```python
from build123d import *

# Parameters (mm, degrees)
BOSS_EXTRUDE1_DEPTH = 20.0000108


with BuildPart() as part:
    # Sketch1 → Boss-Extrude1 (new body)
    with BuildSketch(Plane(origin=(0, 0, 0), x_dir=(1, 0, 0), z_dir=(0, 1, 0))):
        with BuildLine():
            Line((-1.159549536, 2.070936998), (-3.090908521, 3.791368499))
            ThreePointArc((-3.090908521, 3.791368499), (-3.125119474, 3.931396235), (-3.006433754, 4.0132))
            Line((-3.006433754, 4.0132), (-1.7526, 4.0132))
            ThreePointArc((-1.7526, 4.0132), (-1.572994878, 4.087594878), (-1.4986, 4.2672))
            Line((-1.4986, 4.2672), (-1.4986, 4.7498))
            ThreePointArc((-1.4986, 4.7498), (-1.572994878, 4.929405122), (-1.7526, 5.0038))
            Line((-1.7526, 5.0038), (-4.7498, 5.0038))
            ThreePointArc((-4.7498, 5.0038), (-4.929405122, 4.929405122), (-5.0038, 4.7498))
            Line((-5.0038, 4.7498), (-5.0038, 1.7526))
            ThreePointArc((-5.0038, 1.7526), (-4.929405122, 1.572994878), (-4.7498, 1.4986))
            Line((-4.7498, 1.4986), (-4.2672, 1.4986))
            ThreePointArc((-4.2672, 1.4986), (-4.087594878, 1.572994878), (-4.0132, 1.7526))
            Line((-4.0132, 1.7526), (-4.0132, 3.006433754))
            ThreePointArc((-4.0132, 3.006433754), (-3.931396235, 3.125119474), (-3.791368499, 3.090908521))
            Line((-3.791368499, 3.090908521), (-2.070936998, 1.159549536))
            ThreePointArc((-2.070936998, 1.159549536), (-2.023228558, 1.08099247), (-2.0066, 0.9906))
            Line((-2.0066, 0.9906), (-2.0066, 0.7493))
            ThreePointArc((-2.0066, 0.7493), (-1.932205122, 0.569694878), (-1.7526, 0.4953))
            ThreePointArc((-1.7526, 0.4953), (-1.572994878, 0.420905122), (-1.4986, 0.2413))
            Line((-1.4986, 0.2413), (-1.4986, -0.2413))
            ThreePointArc((-1.4986, -0.2413), (-1.572994878, -0.420905122), (-1.7526, -0.4953))
            ThreePointArc((-1.7526, -0.4953), (-1.932205122, -0.569694878), (-2.0066, -0.7493))
            Line((-2.0066, -0.7493), (-2.0066, -0.9906))
            ThreePointArc((-2.0066, -0.9906), (-2.023228558, -1.08099247), (-2.070936998, -1.159549536))
            Line((-2.070936998, -1.159549536), (-3.791368499, -3.090908521))
            ThreePointArc((-3.791368499, -3.090908521), (-3.931396235, -3.125119474), (-4.0132, -3.006433754))
            Line((-4.0132, -3.006433754), (-4.0132, -1.7526))
            ThreePointArc((-4.0132, -1.7526), (-4.087594878, -1.572994878), (-4.2672, -1.4986))
            Line((-4.2672, -1.4986), (-4.7498, -1.4986))
            ThreePointArc((-4.7498, -1.4986), (-4.929405122, -1.572994878), (-5.0038, -1.7526))
            Line((-5.0038, -1.7526), (-5.0038, -4.7498))
            ThreePointArc((-5.0038, -4.7498), (-4.929405122, -4.929405122), (-4.7498, -5.0038))
            Line((-4.7498, -5.0038), (-1.7526, -5.0038))
            ThreePointArc((-1.7526, -5.0038), (-1.572994878, -4.929405122), (-1.4986, -4.7498))
            Line((-1.4986, -4.7498), (-1.4986, -4.2672))
            ThreePointArc((-1.4986, -4.2672), (-1.572994878, -4.087594878), (-1.7526, -4.0132))
            Line((-1.7526, -4.0132), (-3.006433754, -4.0132))
            ThreePointArc((-3.006433754, -4.0132), (-3.125119474, -3.931396235), (-3.090908521, -3.791368499))
            Line((-3.090908521, -3.791368499), (-1.159549536, -2.070936998))
            ThreePointArc((-1.159549536, -2.070936998), (-1.08099247, -2.023228558), (-0.9906, -2.0066))
            Line((-0.9906, -2.0066), (-0.7493, -2.0066))
            ThreePointArc((-0.7493, -2.0066), (-0.569694878, -1.932205122), (-0.4953, -1.7526))
            ThreePointArc((-0.4953, -1.7526), (-0.420905122, -1.572994878), (-0.2413, -1.4986))
            Line((-0.2413, -1.4986), (0.2413, -1.4986))
            ThreePointArc((0.2413, -1.4986), (0.420905122, -1.572994878), (0.4953, -1.7526))
            ThreePointArc((0.4953, -1.7526), (0.569694878, -1.932205122), (0.7493, -2.0066))
            Line((0.7493, -2.0066), (0.9906, -2.0066))
            ThreePointArc((0.9906, -2.0066), (1.08099247, -2.023228558), (1.159549536, -2.070936998))
            Line((1.159549536, -2.070936998), (3.090908521, -3.791368499))
            ThreePointArc((3.090908521, -3.791368499), (3.125119474, -3.931396235), (3.006433754, -4.0132))
            Line((3.006433754, -4.0132), (1.7526, -4.0132))
            ThreePointArc((1.7526, -4.0132), (1.572994878, -4.087594878), (1.4986, -4.2672))
            Line((1.4986, -4.2672), (1.4986, -4.7498))
            ThreePointArc((1.4986, -4.7498), (1.572994878, -4.929405122), (1.7526, -5.0038))
            Line((1.7526, -5.0038), (4.7498, -5.0038))
            ThreePointArc((4.7498, -5.0038), (4.929405122, -4.929405122), (5.0038, -4.7498))
            Line((5.0038, -4.7498), (5.0038, -1.7526))
            ThreePointArc((5.0038, -1.7526), (4.929405122, -1.572994878), (4.7498, -1.4986))
            Line((4.7498, -1.4986), (4.2672, -1.4986))
            ThreePointArc((4.2672, -1.4986), (4.087594878, -1.572994878), (4.0132, -1.7526))
            Line((4.0132, -1.7526), (4.0132, -3.006433754))
            ThreePointArc((4.0132, -3.006433754), (3.931396235, -3.125119474), (3.791368499, -3.090908521))
            Line((3.791368499, -3.090908521), (2.070936998, -1.159549536))
            ThreePointArc((2.070936998, -1.159549536), (2.023228558, -1.08099247), (2.0066, -0.9906))
            Line((2.0066, -0.9906), (2.0066, -0.7493))
            ThreePointArc((2.0066, -0.7493), (1.932205122, -0.569694878), (1.7526, -0.4953))
            ThreePointArc((1.7526, -0.4953), (1.572994878, -0.420905122), (1.4986, -0.2413))
            Line((1.4986, -0.2413), (1.4986, 0.2413))
            ThreePointArc((1.4986, 0.2413), (1.572994878, 0.420905122), (1.7526, 0.4953))
            ThreePointArc((1.7526, 0.4953), (1.932205122, 0.569694878), (2.0066, 0.7493))
            Line((2.0066, 0.7493), (2.0066, 0.9906))
            ThreePointArc((2.0066, 0.9906), (2.023228558, 1.08099247), (2.070936998, 1.159549536))
            Line((2.070936998, 1.159549536), (3.791368499, 3.090908521))
            ThreePointArc((3.791368499, 3.090908521), (3.931396235, 3.125119474), (4.0132, 3.006433754))
            Line((4.0132, 3.006433754), (4.0132, 1.7526))
            ThreePointArc((4.0132, 1.7526), (4.087594878, 1.572994878), (4.2672, 1.4986))
            Line((4.2672, 1.4986), (4.7498, 1.4986))
            ThreePointArc((4.7498, 1.4986), (4.929405122, 1.572994878), (5.0038, 1.7526))
            Line((5.0038, 1.7526), (5.0038, 4.7498))
            ThreePointArc((5.0038, 4.7498), (4.929405122, 4.929405122), (4.7498, 5.0038))
            Line((4.7498, 5.0038), (1.7526, 5.0038))
            ThreePointArc((1.7526, 5.0038), (1.572994878, 4.929405122), (1.4986, 4.7498))
            Line((1.4986, 4.7498), (1.4986, 4.2672))
            ThreePointArc((1.4986, 4.2672), (1.572994878, 4.087594878), (1.7526, 4.0132))
            Line((1.7526, 4.0132), (3.006433754, 4.0132))
            ThreePointArc((3.006433754, 4.0132), (3.125119474, 3.931396235), (3.090908521, 3.791368499))
            Line((3.090908521, 3.791368499), (1.159549536, 2.070936998))
            ThreePointArc((1.159549536, 2.070936998), (1.08099247, 2.023228558), (0.9906, 2.0066))
            Line((0.9906, 2.0066), (0.7493, 2.0066))
            ThreePointArc((0.7493, 2.0066), (0.569694878, 1.932205122), (0.4953, 1.7526))
            ThreePointArc((0.4953, 1.7526), (0.420905122, 1.572994878), (0.2413, 1.4986))
            Line((0.2413, 1.4986), (-0.2413, 1.4986))
            ThreePointArc((-0.2413, 1.4986), (-0.420905122, 1.572994878), (-0.4953, 1.7526))
            ThreePointArc((-0.4953, 1.7526), (-0.569694878, 1.932205122), (-0.7493, 2.0066))
            Line((-0.7493, 2.0066), (-0.9906, 2.0066))
            ThreePointArc((-0.9906, 2.0066), (-1.08099247, 2.023228558), (-1.159549536, 2.070936998))
        make_face()
    extrude(amount=BOSS_EXTRUDE1_DEPTH)


solid = part.part
```
The model under review builds one solid part; all positions refer to its coordinate system, in mm. A direction names the side the tool comes from. Give positions to 0.01 mm unless a question says otherwise; leave off trailing zeros. Loops run counter-clockwise (first coordinate to the right, second up) from the corner with the lowest first, then second, coordinate; pieces in that order, holes last. Notation, with made-up numbers: (22, -28) -> (58, -28) arc R11 ccw to (58, -21) -> close; hole circle Ø5 at (-38, 77.5). An arc over 180 degrees is marked (long way). Use CSV: the item, a comma, the result in double quotes.
1. To check wall thickness, follow probe 1 along Z at (x, y) = (2.25, 8.25); probe 2 along X at (y, z) = (15, -1); probe 3 along X at (y, z) = (3.75, -0.25). State the ranges of each line that lie inside material, in increasing order. Write a range as from..to.
Result:
probe 1,"z = -5..-4.01, -3.04..-1.36, 1.36..3.04, 4.01..5"
probe 2,"x = -2.01..2.01"
probe 3,"x = -1.5..1.5"
2. Consider section A-A, the plane x = -2.75. Write out the cut boundary in (y, z), then the cut area to 3 significant figures.
Result:
outline,"(0, -5) -> (20, -5) -> (20, -4.01) -> (0, -4.01) -> close; (0, -3.49) -> (20, -3.49) -> (20, -1.92) -> (0, -1.92) -> close; (0, 1.92) -> (20, 1.92) -> (20, 3.49) -> (0, 3.49) -> close; (0, 4.01) -> (20, 4.01) -> (20, 5) -> (0, 5) -> close"
area,"102 mm²"
3. Consider section C-C, the plane z = 2.5. Write out the cut boundary in (x, y) (3 decimals).
Result:
outline,"(-5.004, 0) -> (-4.013, 0) -> (-4.013, 20) -> (-5.004, 20) -> close; (-3.265, 0) -> (-1.641, 0) -> (-1.641, 20) -> (-3.265, 20) -> close; (1.641, 0) -> (3.265, 0) -> (3.265, 20) -> (1.641, 20) -> close; (4.013, 0) -> (5.004, 0) -> (5.004, 20) -> (4.013, 20) -> close"
4. Consider section D-D, the plane z = 0. Write out the cut boundary in (x, y).
Result:
outline,"(-1.5, 0) -> (1.5, 0) -> (1.5, 20) -> (-1.5, 20) -> close"
5. For P1, Ø0.5, axis at x = 0, y = 6.5, coming from the -Z side; P2, Ø0.5, axis at x = 0, y = 8, coming from the +Z side, all flat-tipped, find the tip position at first contact; note any pin that passes through.
Result:
P1,"stops at z = -1.5"
P2,"stops at z = 1.5"
6. Consider section B-B, the plane z = -3.5. Write out the cut boundary in (x, y), then the cut area to 3 significant figures.
Result:
outline,"(-5, 0) -> (-2.76, 0) -> (-2.76, 20) -> (-5, 20) -> close; (2.76, 0) -> (5, 0) -> (5, 20) -> (2.76, 20) -> close"
area,"89.6 mm²"
7. The part is to be moulded in two halves that separate along X. For faces 3 (the face through (-3, 10, -5.004)), 4 (the face through (-4.013, 10, 2)), 5 (the face through (-5.004, 10, 3)), say which applies: +X half, -X half, draft (parallel to the pull), parting line (faces both ways), or undercut.
Result:
face 3,"draft"
face 4,"undercut"
face 5,"-X half"
8. Machinability: for faces 1 (the face through (5.004, 10, -3)), 2 (the face through (2.92, 9.86, -2.11)), which of the approach directions +Z, -Z, +X, -X, +Y, -Y give a long, thin tool a straight path to every point of the face, cutting with its end or side? Answer none if there is none.
Result:
face 1,"+Z, -Z, +X, +Y, -Y"
face 2,"+Y, -Y"
